Can you work these out from the model? Positions are in its coordinate system, mm. Give positions to 0.01 mm unless a question says otherwise; leave off trailing zeros. Write each loop counter-clockwise with the first axis right and the second up, starting at its lowest first coordinate (ties: lowest second). Pieces come first, ordered by that corner, then holes. Notation, with made-up numbers: M -36,-9.5 L -32,-9.5 A26 ccw -32,25.5 Z; hole C -23.75,83.5 d2. An arc over 180 degrees is marked long. Use CSV: the item, a comma, the result in double quotes. Start each with the question number.
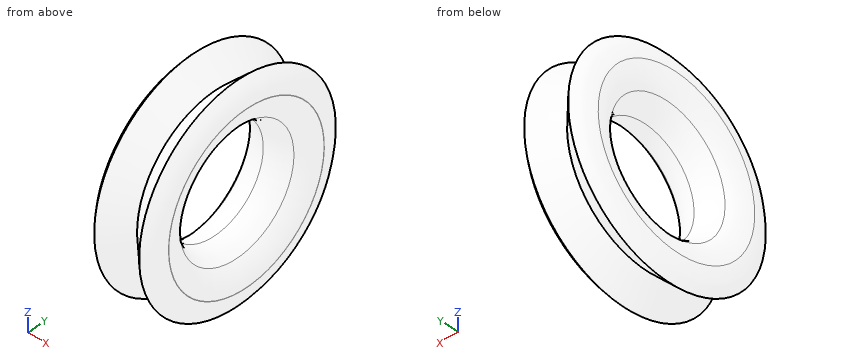
from build123d import *


with BuildPart() as f1:
    # F0 (on Front) → F1 (revolve)
    with BuildSketch(Plane.XZ):
        with BuildLine():
            Line((-3.015464, 28.643063), (-14.102481, 40.005002))
            Line((-14.102481, 40.005002), (-14.29688, 24.131192))
            ThreePointArc((-14.29688, 24.131192), (-8.207439, 25.265121), (-3.015464, 28.643063))
        make_face()
        with BuildLine():
            Line((-14.29688, 24.131192), (-14.102481, 40.005002))
            Line((-14.102481, 40.005002), (-25.464421, 28.917985))
            ThreePointArc((-25.464421, 28.917985), (-20.356727, 25.413908), (-14.29688, 24.131192))
        make_face()
        with BuildLine():
            Line((-29.976291, 40.199401), (-14.102481, 40.005002))
            Line((-14.102481, 40.005002), (-25.189499, 51.366942))
            ThreePointArc((-25.189499, 51.366942), (-28.693576, 46.259247), (-29.976291, 40.199401))
        make_face()
        with BuildLine():
            Line((-25.464421, 28.917985), (-14.102481, 40.005002))
            Line((-14.102481, 40.005002), (-29.976291, 40.199401))
            ThreePointArc((-29.976291, 40.199401), (-28.842362, 34.109959), (-25.464421, 28.917985))
        make_face()
        with BuildLine():
            ThreePointArc((-3.015464, 28.643063), (0.488613, 33.750757), (1.771328, 39.810603))
            Line((1.771328, 39.810603), (-14.102481, 40.005002))
            Line((-14.102481, 40.005002), (-3.015464, 28.643063))
        make_face()
        with BuildLine():
            ThreePointArc((1.771328, 39.810603), (1.772221, 39.907801), (1.772519, 40.005002))
            ThreePointArc((1.772519, 40.005002), (0.601029, 45.990185), (-2.740542, 51.09202))
            Line((-2.740542, 51.09202), (-14.102481, 40.005002))
            Line((-14.102481, 40.005002), (1.771328, 39.810603))
        make_face()
    revolve(axis=Axis((-0.097199, 0, -2.302446), (1, 0, 0)))


solid = f1.part
(1) I want a section at B-B (x = -21.5). Write out the boundary of the cut face in (y, z).
(2) I want a section at C-C (x = -11). Write out the boundary of the cut face in (y, z).
(3) Please list where these lines run through material, in increasing order: L1, parallel to X at y = -30, z = 33; L2, parallel to X at y = 46, z = 4.5; L3, parallel to Z at x = -26.5, y = 11. Write a range as [from, to].
(4) Will these pins go through, and if not, where does the flat tip stop? pin 1 Ø1.5 at (y, z) = (-29.5, 33) entering from -X; pin 2 Ø5 at (x, y) = (-15, 28) entering from +Z; pin 3 Ø6 at (x, z) = (-6.5, 19.5) entering from +Y.
Geometry results:
1,outline,"C 0,-2.3 d99.78; hole C 0,-2.3 d56.52"
2,outline,"C 0,-2.3 d90.67; hole C 0,-2.3 d53.48"
3,L1,"x = [-29.46, -18.03], [-9.98, 1.26]"
3,L2,"x = [-29.41, -18.19], [-9.81, 1.21]"
3,L3,"z = [-53.35, -32.77], [28.16, 48.75]"
4,pin 1,"stops at x = -29.7"
4,pin 2,"stops at z = 34.44"
4,pin 3,"stops at y = 48.19"
